```python
from build123d import *

# Parameters (mm, degrees)
SKETCH1_R                      = 10.75
BOSS_EXTRUDE1_DEPTH            = 2
CUT_EXTRUDE1_REACH             = 4
SKETCH2_R                      = 4
CUT_EXTRUDE1_DIRECTION_2_REACH = 4
SKETCH3_R                      = 20
SKETCH3_R_2                    = 10.75
BOSS_EXTRUDE2_DEPTH            = 9.5
SKETCH6_R                      = 2
CUT_EXTRUDE2_DEPTH             = 20


with BuildPart() as part:
    # Sketch1 → Boss-Extrude1 (new body, symmetric)
    with BuildSketch(Plane.XY):
        with BuildLine():
            Line((-70, -20), (70, -20))
            ThreePointArc((70, -20), (84.142135624, -14.142135624), (90, 0))
            Line((90, 0), (90, 88.85))
            Line((90, 88.85), (-89.389486479, 88.85))
            Line((-89.389486479, 88.85), (-90, 0))
            ThreePointArc((-90, 0), (-84.142135624, -14.142135624), (-70, -20))
        make_face()
        with Locations((70, 0)):
            Circle(SKETCH1_R, mode=Mode.SUBTRACT)
        with Locations((-70, 0)):
            Circle(SKETCH1_R, mode=Mode.SUBTRACT)
    extrude(amount=BOSS_EXTRUDE1_DEPTH, both=True)

    # Cut-Extrude1: up to this face of the body (flat: up to its plane)
    cut_extrude1_end = Plane(part.part.faces().sort_by_distance((0.130461416, 36.187362992, 2))[0])
    # Sketch2 → Cut-Extrude1 (cut, up to the picked face)
    with BuildSketch(Plane.XY, mode=Mode.PRIVATE) as cut_extrude1_sk1:
        with Locations((0.554740673, 69)):
            Circle(SKETCH2_R)
    cut_extrude1_tool1 = split(extrude(cut_extrude1_sk1.sketch, amount=CUT_EXTRUDE1_REACH, mode=Mode.PRIVATE), bisect_by=cut_extrude1_end, keep=Keep.BOTH, mode=Mode.PRIVATE)
    add(cut_extrude1_tool1.solids().sort_by_distance((0.554741, 69, 0))[0], mode=Mode.SUBTRACT)

    # Cut-Extrude1 direction 2: up to this face of the body (flat: up to its plane)
    cut_extrude1_direction_2_end = Plane(part.part.faces().sort_by_distance((0.130461416, 36.187362992, -2))[0])
    # Sketch2 → Cut-Extrude1 direction 2 (cut, up to the picked face)
    with BuildSketch(Plane.XY, mode=Mode.PRIVATE) as cut_extrude1_direction_2_sk1:
        with Locations((0.554740673, 69)):
            Circle(SKETCH2_R)
    cut_extrude1_direction_2_tool1 = split(extrude(cut_extrude1_direction_2_sk1.sketch, amount=-CUT_EXTRUDE1_DIRECTION_2_REACH, mode=Mode.PRIVATE), bisect_by=cut_extrude1_direction_2_end, keep=Keep.BOTH, mode=Mode.PRIVATE)
    add(cut_extrude1_direction_2_tool1.solids().sort_by_distance((0.554741, 69, 0))[0], mode=Mode.SUBTRACT)

    # Sketch3 → Boss-Extrude2 (add, symmetric)
    with BuildSketch(Plane.XY):
        with Locations((-70, 0)):
            Circle(SKETCH3_R)
        with Locations((-70, 0)):
            Circle(SKETCH3_R_2, mode=Mode.SUBTRACT)
        with Locations((70, 0)):
            Circle(SKETCH3_R)
        with Locations((70, 0)):
            Circle(SKETCH3_R_2, mode=Mode.SUBTRACT)
    extrude(amount=BOSS_EXTRUDE2_DEPTH, both=True)

    # Sketch6 → Cut-Extrude2 (cut)
    with BuildSketch(Plane(origin=(0, 0, 0), x_dir=(1, 0, 0), z_dir=(0, 1, 0))):
        with Locations((-70, 0)):
            Circle(SKETCH6_R)
        with Locations((70, 0)):
            Circle(SKETCH6_R)
    extrude(amount=-CUT_EXTRUDE2_DEPTH, mode=Mode.SUBTRACT)


solid = part.part
```
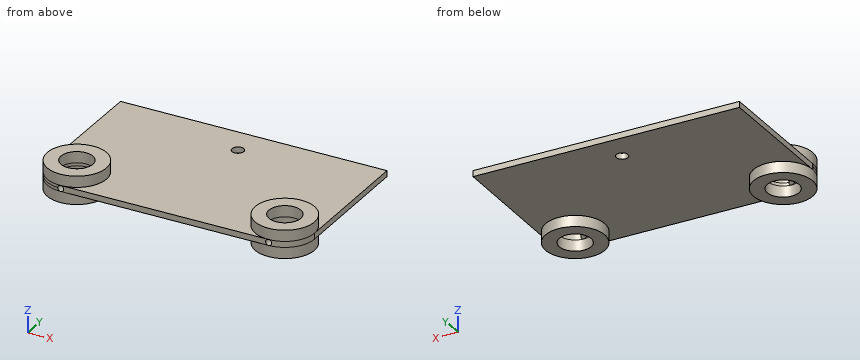
For this review, take the finished solid that the model builds, in its own axes (mm). Give positions to 0.01 mm unless a question says otherwise; leave off trailing zeros. Write each loop counter-clockwise with the first axis right and the second up, starting at its lowest first coordinate (ties: lowest second). Pieces come first, ordered by that corner, then holes. Notation, with made-up numbers: M 61.5,81.25 L 87.5,81.25 A19 ccw 87.5,96.25 Z; hole C -20.5,-27.5 d1. An arc over 180 degrees is marked long. Answer as a JSON object with one key per item and string values. Group by question number.
Item 1: Consider section C-C on x = 53. Write out the cut boundary in (y, z), plus the area to 3 significant figures.
Item 2: Consider section A-A on z = 7.75. Write out the cut boundary in (x, y), plus the area to 3 significant figures.
Item 3: Consider section B-B on y = 69. Write out the cut boundary in (x, z), plus the area to 3 significant figures.
Item 4: Consider section D-D on y = -13. Write out the cut boundary in (x, z).
Item 5: For pin 1 Ø2.5 at (x, z) = (70, 0) entering from -Y; pin 2 Ø1.5 at (x, y) = (-38, 42.5) entering from -Z; pin 3 Ø8 at (x, y) = (23, 72.5) entering from +Z, all flat-tipped, find the tip position at first contact; note any pin that passes through.
Item 6: For probe 1 along X at (y, z) = (0, 6.5); probe 2 along X at (y, z) = (0, -0.95); probe 3 along Z at (x, y) = (-70, -13.75), list the stretches that pass through material, from the lowest coordinate up. Write a range as [from, to].
Check result:
{
 "1": {"outline": "M -20,-2 L -10.54,-2 L -10.54,-9.5 L 10.54,-9.5 L 10.54,-2 L 88.85,-2 L 88.85,2 L 10.54,2 L 10.54,9.5 L -10.54,9.5 L -10.54,2 L -20,2 Z", "area": "751 mm^2"},
 "2": {"outline": "C -70,0 d40; C 70,0 d40; hole C -70,0 d21.5; hole C 70,0 d21.5", "area": "1,790 mm^2"},
 "3": {"outline": "M -89.53,-2 L -3.45,-2 L -3.45,2 L -89.53,2 Z; M 4.55,-2 L 90,-2 L 90,2 L 4.55,2 Z", "area": "686 mm^2"},
 "4": {"outline": "M -85.2,-9.5 L -54.8,-9.5 L -54.8,-2 L 54.8,-2 L 54.8,-9.5 L 85.2,-9.5 L 85.2,9.5 L 54.8,9.5 L 54.8,2 L -54.8,2 L -54.8,9.5 L -85.2,9.5 Z; hole C -70,0 d4; hole C 70,0 d4"},
 "5": {"pin 1": "stops at y = 10.68", "pin 2": "stops at z = -2", "pin 3": "stops at z = 2"},
 "6": {"probe 1": "x = [-90, -80.75], [-59.25, -50], [50, 59.25], [80.75, 90]", "probe 2": "x = [-90, -80.75], [-59.25, 59.25], [80.75, 90]", "probe 3": "z = [-9.5, -2], [2, 9.5]"}
}
